The listing builds one solid part. Answer for the finished solid, in the listing's coordinates (mm). Coordinates: 2 decimals unless noted, no trailing zeros. Order: outer loops, then holes, each group sorted by start corner. A loop starts at its lowest first (then second) coordinate and runs counter-clockwise, first axis right, second up. Notation, with made-up numbers: (-15.75, 6) -> (23.25, 6) arc R4 cw to (23.25, 10) -> close; hole circle Ø10 at (-20, 16.5). An arc over 180 degrees is marked (long way). Write item = value, one per line. Start each with the question number.
```python
from build123d import *

# Parameters (mm, degrees)
RESSALTO_EXTRUS_O5_DEPTH        = 1.25
ESBO_O28_R                      = 1.5
CORTE_EXTRUS_O8_DEPTH           = 3.5
ESBO_O30_OUTSIDE_W              = 14.862
ESBO_O30_OUTSIDE_H              = 14.026
ESBO_O30_OUTSIDE_R              = 2.7
CORTE_EXTRUS_O9_DEPTH           = 3.5
CORTE_EXTRUS_O9_TAPER           = 35
CORTE_EXTRUS_O9_OTHER_WAY_DEPTH = 1
ESBO_O31_OUTSIDE_W              = 13.46
ESBO_O31_OUTSIDE_H              = 12.624
ESBO_O31_OUTSIDE_R              = 2.7
ESBO_O31_OUTSIDE_R_2            = 0.011999843
CORTE_EXTRUS_O10_DEPTH          = 2.5
CORTE_EXTRUS_O10_TAPER          = 35
CHANFRO3_SIZE                   = 0.25


with BuildPart() as part:
    # Esboço2 → Ressalto-extrusão5 (new body, symmetric)
    with BuildSketch(Plane.XY):
        Polygon((3.117691454, 0), (1.558845727, 2.7), (-1.558845727, 2.7), (-3.117691454, 0), (-1.558845727, -2.7), (1.558845727, -2.7), align=None)
    extrude(amount=RESSALTO_EXTRUS_O5_DEPTH, both=True)

    # Esboço28 → Corte-extrusão8 (cut, through all)
    with BuildSketch(Plane.XY.offset(1.25)):
        Circle(ESBO_O28_R)
    extrude(amount=-CORTE_EXTRUS_O8_DEPTH, mode=Mode.SUBTRACT)

    # Esboço30 outside → Corte-extrusão9 (cut)
    with BuildSketch(Plane.XY.offset(1.25)):
        Rectangle(ESBO_O30_OUTSIDE_W, ESBO_O30_OUTSIDE_H)
        Circle(ESBO_O30_OUTSIDE_R, mode=Mode.SUBTRACT)
    extrude(amount=-CORTE_EXTRUS_O9_DEPTH, taper=CORTE_EXTRUS_O9_TAPER, mode=Mode.SUBTRACT)

    # Esboço30 outside → Corte-extrusão9 other way (cut)
    with BuildSketch(Plane.XY.offset(1.25)):
        Rectangle(ESBO_O30_OUTSIDE_W, ESBO_O30_OUTSIDE_H)
        Circle(ESBO_O30_OUTSIDE_R, mode=Mode.SUBTRACT)
    extrude(amount=CORTE_EXTRUS_O9_OTHER_WAY_DEPTH, mode=Mode.SUBTRACT)

    # Esboço31 outside → Corte-extrusão10 (cut)
    with BuildSketch(Plane(origin=(0, 0, -1.25), x_dir=(-1, 0, 0), z_dir=(0, 0, -1))):
        Rectangle(ESBO_O31_OUTSIDE_W, ESBO_O31_OUTSIDE_H)
        Circle(ESBO_O31_OUTSIDE_R, mode=Mode.SUBTRACT)
        with Locations((2.629062893, 0.890906414)):
            Circle(ESBO_O31_OUTSIDE_R_2, mode=Mode.SUBTRACT)
    extrude(amount=-CORTE_EXTRUS_O10_DEPTH, taper=CORTE_EXTRUS_O10_TAPER, mode=Mode.SUBTRACT)

    # Chanfro3
    chanfro3_edges = [part.edges().sort_by_distance(p)[0] for p in [
        (-1.5, 0, -1.25),
        (-1.5, 0, 1.25),
    ]]
    chamfer(chanfro3_edges, length=CHANFRO3_SIZE)


solid = part.part
```
Item 1: Consider probe 1 along Y at (x, z) = (0, -0.6); probe 2 along X at (y, z) = (1, -0.35); probe 3 along X at (y, z) = (-0.9, 0.8). Determine where each line is inside the solid, lowest interval first.
Item 2: Section A-A, the plane z = 0.25 is taken. Give the vertices of the cut face in (x, y).
Item 3: This flat-tipped pin is pushed along its axis until it touches: pin 1 (1.5 mm diameter, centred on y = -1, z = 0, fed in from -X). Where does it stop, or does it pass through?
A:
q1.probe_1 = -2.7 to -1.5, 1.5 to 2.7
q1.probe_2 = -2.54 to -1.12, 1.12 to 2.54
q1.probe_3 = -2.6 to -1.2, 1.2 to 2.6
q2.outline = (-3.12, 0) -> (-1.56, -2.7) -> (1.56, -2.7) -> (3.12, 0) -> (1.56, 2.7) -> (-1.56, 2.7) -> close; hole circle Ø3 at (0, 0)
q3.pin_1 = -2.97
